For this review, take the finished solid that the model builds, in its own axes (mm). A direction names the side the tool comes from. Round coordinates to 2 decimals unless told otherwise and drop trailing zeros. Write each loop counter-clockwise with the first axis right and the second up, starting at its lowest first coordinate (ties: lowest second). Pieces come first, ordered by that corner, then holes. Notation, with made-up numbers: (22, -14) -> (71, -14) arc R32 cw to (71, 14) -> close; hole circle Ø5 at (-7.75, -11). An arc over 180 degrees is marked (long way). Answer as CSV lines item,"result". Start each with the question number.
Item 1: Wall thickness on probe 1 along Y at (x, z) = (0.05, -14.5); probe 2 along X at (y, z) = (-3, 12); probe 3 along X at (y, z) = (1, -12): over which ranges is each line inside the solid? List them lowest first. Write a range as from..to.
Item 2: Take a section at C-C on y = 0. Give the boundary of the cut face in (x, z), then the cut area to 3 significant figures.
Item 3: Take a section at A-A on x = 0. Give the boundary of the cut face in (y, z).
Item 4: Mouldability with a two-part tool opening along X and no side actions: class faces 1 (the flat face through (0, 0, 7.5)), 2 (the flat face through (2.5, 0, -9)), 3 (the cylindrical face through (5, 0, 14)), 4 (the flat face through (-3.25, 2, 12)) as +X half, -X half, draft (parallel to the pull), parting line (faces both ways), or undercut.
Item 5: Take a section at D-D on z = -14.5. Give the boundary of the cut face in (x, y), then the cut area to 3 significant figures.
Item 6: Take a section at B-B on z = 12.5. Give the boundary of the cut face in (x, y), then the cut area to 3 significant figures.
Item 7: For pin 1 Ø4 at (x, y) = (-3.5, 1.5) entering from -Z; pin 2 Ø1.8 at (y, z) = (0, 12.5) entering from -X; pin 3 Ø1 at (x, y) = (3.5, 1) entering from -Z; pin 4 Ø3.5 at (y, z) = (0, -14.5) entering from -X, all flat-tipped, find the tip position at first contact; note any pin that passes through.
Item 8: Machinability: for faces 5 (the flat face through (-2.5, 0, -9)), 6 (the flat face through (6, 0, 9)), 7 (the flat face through (4, 0, 0)), which of the approach directions +Z, -Z, +X, -X, +Y, -Y give a long, thin tool a straight path to every point of the face, cutting with its end or side? Answer none if there is none.
```python
from build123d import *
from build123d.topology import SkipClean

# Parameters (mm, degrees)
SALIENTE_EXTRUIR1_DEPTH    = 2.5
CORTAR_EXTRUIR1_DEPTH      = 19.020821291
CORTAR_EXTRUIR1_DEPTH_BACK = 19.020821291
CROQUIS2_R                 = 1.5
CROQUIS3_R                 = 1.5
SALIENTE_EXTRUIR2_DEPTH    = 6
CORTAR_EXTRUIR2_DEPTH      = 3.25


with BuildPart() as part:
    # Croquis1 → Saliente-Extruir1 (new, symmetric)
    with BuildSketch(Plane(origin=(0, 0, 0), x_dir=(0, 0, -1), z_dir=(1, 0, 0))):
        with BuildLine():
            Line((-16.5, 3.5), (16.5, 3.5))
            ThreePointArc((16.5, 3.5), (17.207106781, 3.207106781), (17.5, 2.5))
            Line((17.5, 2.5), (17.5, -2.5))
            ThreePointArc((17.5, -2.5), (17.207106781, -3.207106781), (16.5, -3.5))
            Line((16.5, -3.5), (-16.5, -3.5))
            ThreePointArc((-16.5, -3.5), (-17.207106781, -3.207106781), (-17.5, -2.5))
            Line((-17.5, -2.5), (-17.5, 2.5))
            ThreePointArc((-17.5, 2.5), (-17.207106781, 3.207106781), (-16.5, 3.5))
        make_face()
    extrude(amount=SALIENTE_EXTRUIR1_DEPTH, both=True)

    # Croquis2 → Cortar-Extruir1 (cut, two sides: drawn at the far end of the back side and taken through both)
    with BuildSketch(Plane(origin=(0, 0, 0), x_dir=(0, 0, -1), z_dir=(1, 0, 0)).offset(-CORTAR_EXTRUIR1_DEPTH_BACK)):
        with Locations((-12.5, 0)):
            Circle(CROQUIS2_R)
        with Locations((14.5, 0)):
            Circle(CROQUIS2_R)
    extrude(amount=CORTAR_EXTRUIR1_DEPTH + CORTAR_EXTRUIR1_DEPTH_BACK, mode=Mode.SUBTRACT)

    # Croquis3 → Saliente-Extruir2 (add, symmetric)
    with SkipClean():  # the faces are left unmerged after this step: merging them gives an invalid solid
        with BuildSketch(Plane(origin=(0, 0, 0), x_dir=(0, 0, -1), z_dir=(1, 0, 0))):
            with BuildLine():
                Line((-17.5, 2.5), (-17.5, -2.5))
                ThreePointArc((-17.5, -2.5), (-17.207106781, -3.207106781), (-16.5, -3.5))
                Line((-16.5, -3.5), (0, -3.5))
                Line((0, -3.5), (0, 3.5))
                Line((0, 3.5), (-16.5, 3.5))
                ThreePointArc((-16.5, 3.5), (-17.207106781, 3.207106781), (-17.5, 2.5))
            make_face()
            with Locations((-12.5, 0)):
                Circle(CROQUIS3_R, mode=Mode.SUBTRACT)
        extrude(amount=SALIENTE_EXTRUIR2_DEPTH, both=True)
    add(part.part.scale(1), mode=Mode.REPLACE)  # the faces are merged on a copy

    # Croquis4 → Cortar-Extruir2 (cut, symmetric)
    with BuildSketch(Plane(origin=(0, 0, 0), x_dir=(0, 0, -1), z_dir=(1, 0, 0))):
        with BuildLine():
            Line((-16.5, 3.5), (-7.5, 3.5))
            Line((-7.5, 3.5), (-7.5, -3.5))
            Line((-7.5, -3.5), (-16.5, -3.5))
            ThreePointArc((-16.5, -3.5), (-17.207106781, -3.207106781), (-17.5, -2.5))
            Line((-17.5, -2.5), (-17.5, 2.5))
            ThreePointArc((-17.5, 2.5), (-17.207106781, 3.207106781), (-16.5, 3.5))
        make_face()
    extrude(amount=CORTAR_EXTRUIR2_DEPTH, both=True, mode=Mode.SUBTRACT)


solid = part.part
```
Output values:
1,probe 1,"y = -3.5..-1.5, 1.5..3.5"
1,probe 2,"x = -6..-3.25, 3.25..6"
1,probe 3,"x = -2.5..2.5"
2,outline,"(-6, 0) -> (-2.5, 0) -> (-2.5, -13) -> (2.5, -13) -> (2.5, 0) -> (6, 0) -> (6, 11) -> (3.25, 11) -> (3.25, 7.5) -> (-3.25, 7.5) -> (-3.25, 11) -> (-6, 11) -> close; (-6, 14) -> (-3.25, 14) -> (-3.25, 17.5) -> (-6, 17.5) -> close; (-2.5, -17.5) -> (2.5, -17.5) -> (2.5, -16) -> (-2.5, -16) -> close; (3.25, 14) -> (6, 14) -> (6, 17.5) -> (3.25, 17.5) -> close"
2,area,"201 mm^2"
3,outline,"(-3.5, -16.5) arc R1 ccw to (-2.5, -17.5) -> (2.5, -17.5) arc R1 ccw to (3.5, -16.5) -> (3.5, 7.5) -> (-3.5, 7.5) -> close; hole circle Ø3 at (0, -14.5)"
4,face 1,"undercut"
4,face 2,"+X half"
4,face 3,"draft"
4,face 4,"undercut"
5,outline,"(-2.5, -3.5) -> (2.5, -3.5) -> (2.5, -1.5) -> (-2.5, -1.5) -> close; (-2.5, 1.5) -> (2.5, 1.5) -> (2.5, 3.5) -> (-2.5, 3.5) -> close"
5,area,"20.0 mm^2"
6,outline,"(-6, -3.5) -> (-3.25, -3.5) -> (-3.25, -1.5) -> (-6, -1.5) -> close; (-6, 1.5) -> (-3.25, 1.5) -> (-3.25, 3.5) -> (-6, 3.5) -> close; (3.25, -3.5) -> (6, -3.5) -> (6, -1.5) -> (3.25, -1.5) -> close; (3.25, 1.5) -> (6, 1.5) -> (6, 3.5) -> (3.25, 3.5) -> close"
6,area,"22.0 mm^2"
7,pin 1,"stops at z = -17.5"
7,pin 2,"passes through"
7,pin 3,"stops at z = 0"
7,pin 4,"stops at x = -2.5"
8,face 5,"-Z, -X, +Y, -Y"
8,face 6,"+Z, -Z, +X, +Y, -Y"
8,face 7,"-Z, +X, +Y, -Y"
